Input: part model. Units: mm. Frame: model coordinates. A direction names the side the tool comes from. Coordinates: 2 decimals unless noted, no trailing zeros. Order: outer loops, then holes, each group sorted by start corner. A loop starts at its lowest first (then second) coordinate and runs counter-clockwise, first axis right, second up. Notation, with made-up numbers: (2.25, -31.75) -> (41.25, -31.75) arc R20 ccw to (41.25, -21.75) -> close; hole circle Ø7 at (-28.5, 14.25). An arc over 180 degrees is marked (long way). Answer as CSV lines item,"result".
from build123d import *

# Parameters (mm, degrees)
F2_R     = 50.8
F4_DEPTH = 6.35
F5_R     = 19.05
F5_R_2   = 12.7
F6_DEPTH = 38.1
F3_R     = 50.8
F7_DEPTH = 6.35


with BuildPart() as f4:
    # F2 (on offset) → F4 (new body)
    with BuildSketch(Plane.YZ.offset(-38.1)):
        Circle(F2_R)
    extrude(amount=-F4_DEPTH)

    # F5 (on Right) → F6 (join, symmetric)
    with BuildSketch(Plane.YZ):
        Circle(F5_R)
        Circle(F5_R_2, mode=Mode.SUBTRACT)
    extrude(amount=F6_DEPTH, both=True)

    # F3 (on offset) → F7 (join)
    with BuildSketch(Plane.YZ.offset(38.1)):
        Circle(F3_R)
    extrude(amount=F7_DEPTH)


solid = f4.part
1. Ray query, line 1 along Z through (x, y) = (15, 0); line 2 along X through (y, z) = (-1, 4.5); line 3 along Z through (x, y) = (-16.5, 3). Return the intervals inside material, ascending.
Findings:
line 1,"z = -19.05 to -12.7, 12.7 to 19.05"
line 2,"x = -44.45 to -38.1, 38.1 to 44.45"
line 3,"z = -18.81 to -12.34, 12.34 to 18.81"
2. Cut plane D-D (x = 24). Return the cut outline in (y, z).
Findings:
outline,"circle Ø38.1 at (0, 0); hole circle Ø25.4 at (0, 0)"
3. Reachability of faces 4 (the face through (38.1, 22, 1)), 5 (the face through (-41.231, -11.012, -49.592)) from +Z, -Z, +X, -X, +Y, -Y: full face, straight path, thin tool, end or side. Return the list, or none.
Findings:
face 4,"none"
face 5,"+X, -X"
4. Contact query for flat-ended pins moving along their axis: pin 1 (1.5 mm diameter, centred on x = 0.5, z = -16, fed in from +Y); pin 2 (1.5 mm diameter, centred on x = 2.5, z = 4, fed in from +Y); pin 3 (12 mm diameter, centred on x = 17.5, z = 12, fed in from +Y). Output: stop coordinate, or through.
Findings:
pin 1,"stops at y = 11.42"
pin 2,"stops at y = 18.77"
pin 3,"stops at y = 18.08"
5. Cut plane A-A (y = 0). Return the cut outline in (x, z).
Findings:
outline,"(-44.45, -50.8) -> (-38.1, -50.8) -> (-38.1, -19.05) -> (38.1, -19.05) -> (38.1, -50.8) -> (44.45, -50.8) -> (44.45, 50.8) -> (38.1, 50.8) -> (38.1, 19.05) -> (-38.1, 19.05) -> (-38.1, 50.8) -> (-44.45, 50.8) -> close; hole (-38.1, -12.7) -> (38.1, -12.7) -> (38.1, 12.7) -> (-38.1, 12.7) -> close"
6. Mould query, pull axis Z, two halves, no side actions, for faces 1 (the face through (0.53, -15.12, -11.59)), 2 (the face through (38.1, 0, 0)), 3 (the face through (-44.45, -1, 1)). Classes: released by +Z, released by -Z, zero draft, split by the parting line, or undercut.
Findings:
face 1,"split by the parting line"
face 2,"undercut"
face 3,"zero draft"
7. Cut plane C-C (y = -42). Return the cut outline in (x, z), plus the area to 3 significant figures.
Findings:
outline,"(-44.45, -28.58) -> (-38.1, -28.58) -> (-38.1, 28.58) -> (-44.45, 28.58) -> close; (38.1, -28.58) -> (44.45, -28.58) -> (44.45, 28.58) -> (38.1, 28.58) -> close"
area,"726 mm2"
